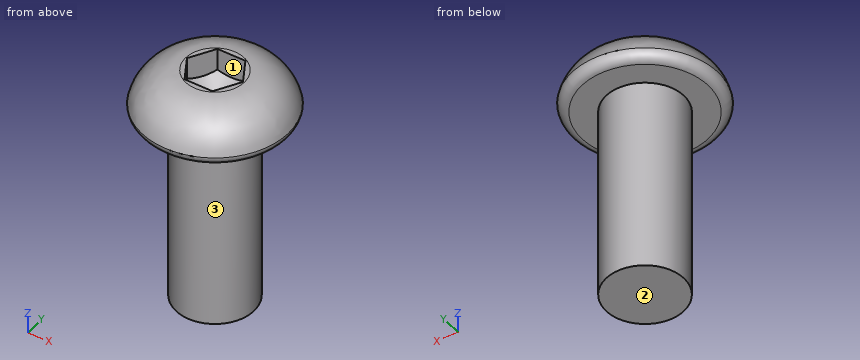
Autodesk Inventor part; units mm, degrees
ref_plane "YZ Plane" through (0, 0, 0) normal (1, 0, 0) x (0, 1, 0)
ref_plane "XZ Plane" through (0, 0, 0) normal (0, 1, 0) x (-1, 0, 0)
ref_plane "XY Plane" through (0, 0, 0) normal (0, 0, 1) x (1, 0, 0)
sketch "Sketch1" plane through (0, 0, 0) normal (0, 0, 1) x (1, 0, 0)
  circle A0 centre (0, 0) radius 3.75
  dimension "d0" = 7.5
extrude "Extrusion1" add sketch "Sketch1" along normal blind 2.3
fillet "Fillet3" radius 0.5 1 edges at (-3.75, 0, 0)
fillet "Fillet4" radius 2.3 1 edges at (-3.75, 0, 2.3)
sketch "草圖6" plane through (0, 0, 2.3) normal (0, 0, 1) x (1, 0, 0)
  circle A0 centre (0, 0) radius 1.505
  line L0 (0.7217, 1.25) -> (1.4434, 0)
  line L1 (1.4434, 0) -> (0.7217, -1.25)
  line L2 (0.7217, -1.25) -> (-0.7217, -1.25)
  line L3 (-0.7217, -1.25) -> (-1.4434, 0)
  line L4 (-1.4434, 0) -> (-0.7217, 1.25)
  line L5 (-0.7217, 1.25) -> (0.7217, 1.25)
  dimension "d27" = 2.5
extrude "擠出4" cut sketch "草圖6" against normal blind 2 contours L0 L1 L2 L3 L4 L5
sketch "草圖7" plane through (0, 0, 0) normal (1, 0, 0) x (0, 1, 0)
  line L0 (0, 0.3) -> (-2, 1.5017)
  line L1 (-2, 1.5017) -> (-2, 0.3)
  line L2 (0, 0.3) -> (-2, 0.3)
  line L3 (0, 0) -> (0, 2.4201)
  dimension "d30" = 0.3
  dimension "d31" = 31
  dimension "d34" = 2
revolve "迴轉3" add sketch "草圖7" angle 360 about axis through (0, 0, 0) along (0, 0, 1)
sketch "草圖8" plane through (0, 0, 0) normal (0, 0, -1) x (-1, 0, 0)
  circle A0 centre (0, 0) radius 3.25
  circle A1 centre (0, 0) radius 2
  dimension "d35" = 4
extrude "擠出5" add sketch "草圖8" along normal blind 10 contours A1
thread "螺紋2"
properties part number "screw_M3_10_hex"
The listing builds one solid part. Answer for the finished solid, in the listing's coordinates (mm). Face numbers are marked on the shaded views. A direction names the side the tool comes from. Give positions to 0.01 mm unless a question says otherwise; leave off trailing zeros. Loops run counter-clockwise (first coordinate to the right, second up) from the corner with the lowest first, then second, coordinate; pieces in that order, holes last. Notation, with made-up numbers: (19, 68) - (73, 68) arc R11 ccw to (73, 76) - close; hole circle Ø3 at (43, -35). An arc over 180 degrees is marked (long way). Return JSON: item names as keys, results as strings. Group by question number.
1. Straight lines are drawn through the part: line 1 (Z direction, x = -1.25, y = -1); line 2 (X direction, y = 0.5, z = -3.25); line 3 (Y direction, x = 1.5, z = -0.5). For each, find the intervals that lie inside material, in ascending order. Write a range as [from, to].
2. Given pin 1 Ø3 at (x, z) = (-1, -6) entering from +Y; pin 2 Ø4 at (x, z) = (-2.5, -4) entering from +Y; pin 3 Ø1.4 at (x, z) = (0, 1.5) entering from -Y, each flat-ended and moving along its own axis, determine where each tip first touches the part or whether it passes through.
3. Find section A-A (z = -1). Write down the section's boundary in (x, y).
4. Which of the six approach directions +Z, -Z, +X, -X, +Y, -Y give full straight-line access (tool end or side, diameter ignored) to the marked faces 1, 2 and 3?
Verdict:
{
 "1": {"line 1": "z = [-10, 2.3]", "line 2": "x = [-1.94, 1.94]", "line 3": "y = [-1.32, 1.32]"},
 "2": {"pin 1": "stops at y = 2", "pin 2": "stops at y = 1.94", "pin 3": "stops at y = -3.66"},
 "3": {"outline": "circle Ø4 at (0, 0)"},
 "4": {"face 1": "+Z", "face 2": "-Z, +X, -X, +Y, -Y", "face 3": "-Z"}
}
